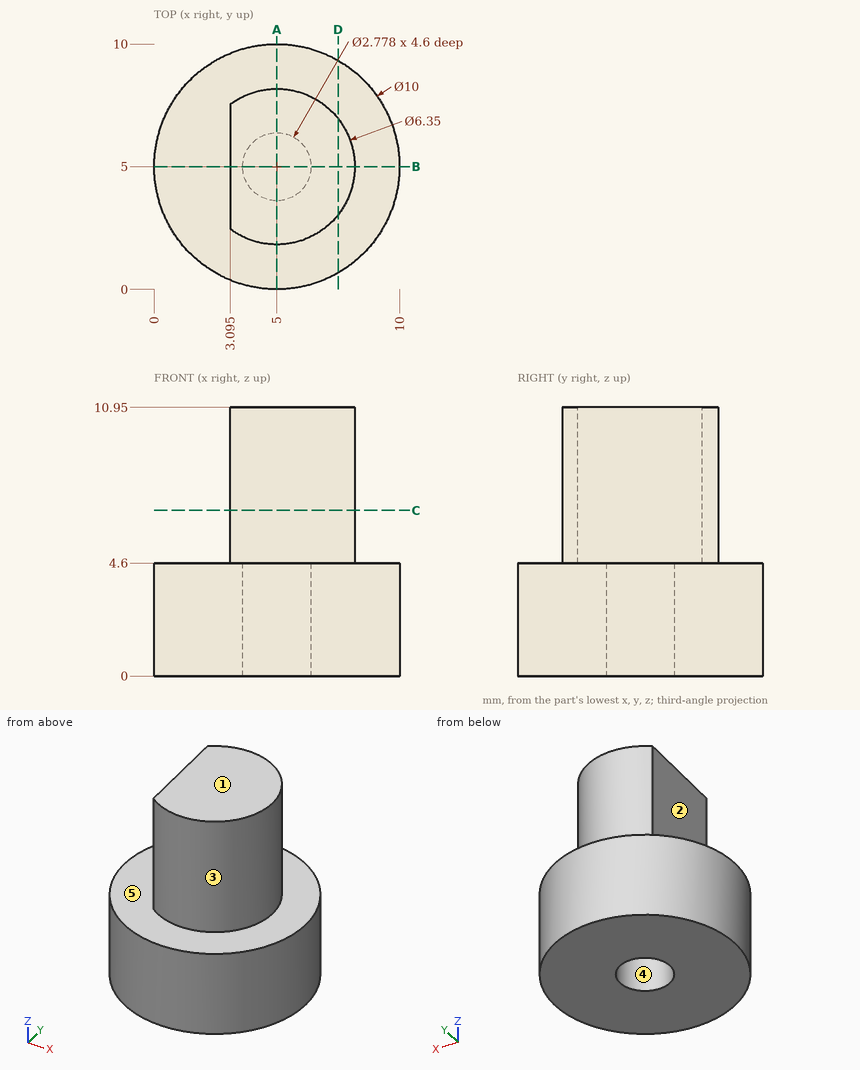
Design review of the part shown in the three views and the two pictorial views. Dimensions are in mm from the part's minimum x, y and z. A direction names the side the tool comes from. Round coordinates to 2 decimals unless told otherwise and drop trailing zeros. Write each loop counter-clockwise with the first axis right and the second up, starting at its lowest first coordinate (ties: lowest second). Pieces come first, ordered by that corner, then holes.
1) Machinability: for the marked faces 1 and 2, which of the approach directions +Z, -Z, +X, -X, +Y, -Y give a long, thin tool a straight path to every point of the face, cutting with its end or side? Answer none if there is none.
Answer below:
face 1: +Z, +X, -X, +Y, -Y
face 2: +Z, -X, +Y, -Y
2) Take a section at A-A on x = 5. Give the boundary of the cut face in (y, z) (3 decimals).
Answer below:
outline: (0, 0) - (3.611, 0) - (3.611, 4.6) - (6.389, 4.6) - (6.389, 0) - (10, 0) - (10, 4.6) - (8.175, 4.6) - (8.175, 10.95) - (1.825, 10.95) - (1.825, 4.6) - (0, 4.6) - close
3) Insertion check: pin 1 Ø1.7 at (x, y) = (5, 5) entering from -Z; pin 2 Ø1.5 at (x, y) = (2, 7) entering from +Z; pin 3 Ø4 at (y, z) = (4.5, 8) entering from -X (3 decimals). Each pin has a flat end and moves straight along its axis. Give the tip position at first contact, or say it passes through.
Answer below:
pin 1: stops at z = 4.6
pin 2: stops at z = 4.6
pin 3: stops at x = 3.095
4) Mouldability with a two-part tool opening along X and no side actions: class the marked faces 3, 4 and 5 as +X half, -X half, draft (parallel to the pull), parting line (faces both ways), or undercut.
Answer below:
face 3: parting line
face 4: undercut
face 5: draft
5) Take a section at C-C on z = 6.75. Give the boundary of the cut face in (x, y) (3 decimals), then the cut area to 3 significant figures.
Answer below:
outline: (3.095, 2.46) arc R3.175 ccw (long way) to (3.095, 7.54) - close
area: 27.2 mm2
6) Take a section at D-D on x = 7.5. Give the boundary of the cut face in (y, z), then the cut area to 3 significant figures.
Answer below:
outline: (0.67, 0) - (9.33, 0) - (9.33, 4.6) - (6.96, 4.6) - (6.96, 10.95) - (3.04, 10.95) - (3.04, 4.6) - (0.67, 4.6) - close
area: 64.7 mm2
7) Take a section at B-B on y = 5. Give the boundary of the cut face in (x, z) (3 decimals), then the cut area to 3 significant figures.
Answer below:
outline: (0, 0) - (3.611, 0) - (3.611, 4.6) - (6.389, 4.6) - (6.389, 0) - (10, 0) - (10, 4.6) - (8.175, 4.6) - (8.175, 10.95) - (3.095, 10.95) - (3.095, 4.6) - (0, 4.6) - close
area: 65.5 mm2
8) For line 1 along Y through (x, z) = (5, 2.2); line 2 along Y through (x, z) = (5.75, 4.25); line 3 along Z through (x, y) = (0.5, 5), list the stretches that pass through material, from the lowest coordinate up.
Answer below:
line 1: y = 0 to 3.61, 6.39 to 10
line 2: y = 0.06 to 3.83, 6.17 to 9.94
line 3: z = 0 to 4.6
